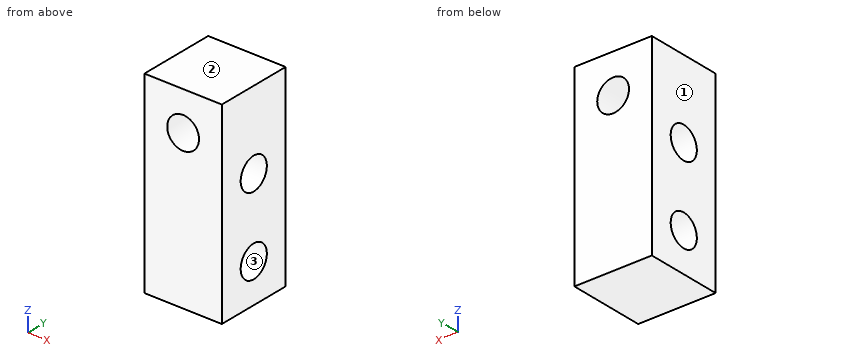
```python
from build123d import *

# Parameters (mm, degrees)
SKETCH_W        = 20
SKETCH_H        = 20
PAD_DEPTH       = 50
SKETCH001_R     = 4.1
POCKET_DEPTH    = 20
SKETCH002_R     = 4.1
POCKET001_DEPTH = 20


with BuildPart() as part:
    # Sketch → Pad (new body)
    with BuildSketch(Plane.XY):
        with Locations((-13.292078, 23.65859)):
            Rectangle(SKETCH_W, SKETCH_H)
    extrude(amount=PAD_DEPTH)

    # Sketch001 → Pocket (cut)
    with BuildSketch(Plane.YZ.offset(-3.292078)):
        with Locations((23.65859, 10)):
            Circle(SKETCH001_R)
        with Locations((23.65859, 30)):
            Circle(SKETCH001_R)
    extrude(amount=-POCKET_DEPTH, mode=Mode.SUBTRACT)

    # Sketch002 → Pocket001 (cut)
    with BuildSketch(Plane.XZ.offset(-13.65859)):
        with Locations((-13.292078, 40)):
            Circle(SKETCH002_R)
    extrude(amount=-POCKET001_DEPTH, mode=Mode.SUBTRACT)


solid = part.part
```
Verification items for the finished model (mm, model axes). Face numbers are marked on the shaded views. Give positions to 0.01 mm unless a question says otherwise; leave off trailing zeros. Order: outer loops, then holes, each group sorted by start corner. A loop starts at its lowest first (then second) coordinate and runs counter-clockwise, first axis right, second up. Notation, with made-up numbers: M 38,-22.75 L 66,-22.75 A36 ccw 66,14.25 Z; hole C 4.25,-15.75 d5. An arc over 180 degrees is marked long. Return JSON: item names as keys, results as strings. Group by question number.
1) Section check B-B on y = 21.5. Record the cut outline in (x, z).
2) Section check D-D on y = 32. Record the cut outline in (x, z).
3) Section check C-C on x = -18.5. Record the cut outline in (y, z).
4) Go/stop test with a flat-tipped pin: pin 1 Ø7.5 at (y, z) = (23.66, 10) entering from +X. Record where the tip stops, or that it passes through.
5) Section check A-A on z = 40. Record the cut outline in (x, y), and give its area (3 significant figures).
6) Scan lines: line 1 (Z direction, x = -11, y = 27); line 2 (Z direction, x = -15.5, y = 26.5); line 3 (Z direction, x = -21.5, y = 23). Record each from-to range of solid material in increasing order.
7) Mould release check, pull along Z, two halves, no side actions. Record for the marked faces 1, 2 and 3: pulls with the +Z half, pulls with the -Z half, needs draft (parallel to the pull), parting line crosses it, or undercut.
Answer block:
{
 "1": {"outline": "M -23.29,0 L -3.29,0 L -3.29,6.51 L -23.29,6.51 Z; M -23.29,13.49 L -3.29,13.49 L -3.29,26.51 L -23.29,26.51 Z; M -23.29,33.49 L -3.29,33.49 L -3.29,50 L -23.29,50 Z; hole C -13.29,40 d8.2"},
 "2": {"outline": "M -23.29,0 L -3.29,0 L -3.29,50 L -23.29,50 Z; hole C -13.29,40 d8.2"},
 "3": {"outline": "M 13.66,0 L 33.66,0 L 33.66,50 L 13.66,50 Z; hole C 23.66,10 d8.2; hole C 23.66,30 d8.2"},
 "4": {"pin 1": "passes through"},
 "5": {"outline": "M -23.29,13.66 L -17.39,13.66 L -17.39,33.66 L -23.29,33.66 Z; M -9.19,13.66 L -3.29,13.66 L -3.29,33.66 L -9.19,33.66 Z", "area": "236 mm^2"},
 "6": {"line 1": "z = 0 to 7.62, 12.38 to 27.62, 32.38 to 36.6, 43.4 to 50", "line 2": "z = 0 to 7.04, 12.96 to 27.04, 32.96 to 36.55, 43.45 to 50", "line 3": "z = 0 to 5.95, 14.05 to 25.95, 34.05 to 50"},
 "7": {"face 1": "needs draft", "face 2": "pulls with the +Z half", "face 3": "undercut"}
}
